Geometry check sheet. Reference: the model listing, model coordinates, mm. Coordinates: 2 decimals unless noted, no trailing zeros.
Autodesk Inventor part; units mm, degrees
ref_plane "YZ Plane" through (0, 0, 0) normal (1, 0, 0) x (0, 1, 0)
ref_plane "XZ Plane" through (0, 0, 0) normal (0, 1, 0) x (-1, 0, 0)
ref_plane "XY Plane" through (0, 0, 0) normal (0, 0, 1) x (1, 0, 0)
sketch "Sketch1" plane through (0, 0, 0) normal (0, 0, 1) x (1, 0, 0)
  line L0 (-28, 61) -> (-28, 11)
  arc A0 (-28, 61) -> (-31, 64) centre (-31, 61) ccw
  line L1 (-110, 64) -> (-31, 64)
  arc A1 (-110, 64) -> (-113, 61) centre (-110, 61) ccw
  line L2 (-113, 11) -> (-113, 61)
  arc A2 (-113, 11) -> (-110, 8) centre (-110, 11) ccw
  line L3 (-31, 8) -> (-110, 8)
  arc A3 (-31, 8) -> (-28, 11) centre (-31, 11) ccw
  circle A4 centre (-89.5855, 11.5) radius 1.3645
  circle A5 centre (-89.5855, 60.5) radius 1.3645
  circle A6 centre (-31.5, 60.5) radius 1.3645
  circle A7 centre (-31.5, 11.5) radius 1.3645
  circle A8 centre (-31.4673, 17.5489) radius 1.5
  circle A9 centre (-89.237, 54.3009) radius 1.5
  point P0 (0, 0)
extrude "Extrusion1" add sketch "Sketch1" along normal blind 59
properties part number "UPSboard"
1. Gauge pin test, flat end, axial feed: pin 1 Ø1.8 at (x, y) = (-89.24, 54.3) entering from +Z. Record the tip position at first contact, or that the pin passes through.
Computed values:
pin 1: passes through
2. Thickness scan on line 1 along Y through (x, z) = (-31.5, 40); line 2 along X through (y, z) = (60, 35); line 3 along Y through (x, z) = (-31, 47). Record the ranges inside material, lowest first.
Computed values:
line 1: y = 8 to 10.14, 12.86 to 16.05, 19.05 to 59.14, 61.86 to 64
line 2: x = -113 to -90.86, -88.32 to -32.77, -30.23 to -28
line 3: y = 8 to 10.23, 12.77 to 16.12, 18.97 to 59.23, 61.77 to 64
3. Draft check along Y on faces 1 (the cylindrical face through (-30.87, 12.71, 29.09)), 2 (the cylindrical face through (-112.1, 8.86, 29.09)), 3 (the cylindrical face through (-112.14, 63.1, 29.09)), 4 (the flat face through (-28, 36, 29)). Enter one of: released by +Y, released by -Y, zero draft, split by the parting line, or undercut.
Computed values:
face 1: undercut
face 2: released by -Y
face 3: released by +Y
face 4: zero draft
